Read the model definition and answer for the solid it produces. Units are mm, in the model's axes. Coordinates: 2 decimals unless noted, no trailing zeros. Loops run counter-clockwise (first coordinate to the right, second up) from the corner with the lowest first, then second, coordinate; pieces in that order, holes last. Notation, with made-up numbers: (59.5, 14.5) -> (67.5, 14.5) arc R31 ccw to (67.5, 38.5) -> close; hole circle Ø10 at (-5.5, 67.5). An arc over 180 degrees is marked (long way). Answer as CSV lines item,"result".
```python
from build123d import *

# Parameters (mm, degrees)
EXTRUDE_1_DEPTH     = 4
SKETCH_3_R          = 15
SKETCH_3_R_2        = 2.1
CUT_EXTRUDE_1_DEPTH = 4
SKETCH_4_R          = 2.15
CUT_EXTRUDE_2_DEPTH = 4
SKETCH_5_R          = 1.6
CUT_EXTRUDE_3_DEPTH = 4
EXTRUDE_2_DEPTH     = 4


with BuildPart() as part:
    # 草图2 → 凸台-拉伸1 (new body)
    with BuildSketch(Plane.XY):
        Polygon((131.137809217, 89.374251193), (132.400858097, 9.374251193), (72.408334633, 8.427082574), (71.145285753, 88.427082574), align=None)
    extrude(amount=EXTRUDE_1_DEPTH)

    # 草图3 → 切除-拉伸1 (cut)
    with BuildSketch(Plane.XY.offset(4)):
        with Locations((100.473333038, 48.885132061)):
            Circle(SKETCH_3_R)
        with Locations((119.759256959, 54.181653421)):
            Circle(SKETCH_3_R_2)
        with Locations((95.417293127, 29.53477133)):
            Circle(SKETCH_3_R_2)
        with Locations((86.243449028, 62.938971432)):
            Circle(SKETCH_3_R_2)
    extrude(amount=-CUT_EXTRUDE_1_DEPTH, mode=Mode.SUBTRACT)

    # 草图4 → 切除-拉伸2 (cut)
    with BuildSketch(Plane.XY.offset(4)):
        with Locations((77.239254962, 82.522547089)):
            Circle(SKETCH_4_R)
        with Locations((78.31271273, 14.531020496)):
            Circle(SKETCH_4_R)
    extrude(amount=-CUT_EXTRUDE_2_DEPTH, mode=Mode.SUBTRACT)

    # 草图5 → 切除-拉伸3 (cut)
    with BuildSketch(Plane.XY.offset(4)):
        with Locations((120.233896778, 83.201351266)):
            Circle(SKETCH_5_R)
        with Locations((120.423330501, 71.202846573)):
            Circle(SKETCH_5_R)
        with Locations((121.117920822, 27.208329366)):
            Circle(SKETCH_5_R)
        with Locations((121.307354546, 15.209824673)):
            Circle(SKETCH_5_R)
    extrude(amount=-CUT_EXTRUDE_3_DEPTH, mode=Mode.SUBTRACT)

    # 草图6 → 凸台-拉伸2 (add)
    with BuildSketch(Plane.XY.offset(4)):
        Polygon((132.156015483, 24.882288469), (131.934981929, 38.882288469), (135.934483494, 38.945433043), (136.155517047, 24.945433043), align=None)
        Polygon((131.603500455, 59.877927156), (131.382494444, 73.876182631), (135.381996008, 73.939327206), (135.60300202, 59.941071731), align=None)
    extrude(amount=-EXTRUDE_2_DEPTH)


solid = part.part
```
Q1. Given pin 1 Ø2.5 at (x, y) = (77.24, 82.52) entering from -Z; pin 2 Ø1 at (y, z) = (39.5, 1) entering from -X, each flat-ended and moving along its own axis, determine where each tip first touches the part or whether it passes through.
Results:
pin 1,"passes through"
pin 2,"stops at x = 71.91"
Q2. For a pull along X with two mould halves and no side action, classify faces 1 (the face through (119, 49, 0)), 2 (the face through (119.52, 27.28, 2.03)) as pulls with the +X half, pulls with the -X half, needs draft (parallel to the pull), parting line crosses it, or undercut.
Results:
face 1,"needs draft"
face 2,"undercut"
Q3. Find the intervals of material crossed by probe 1 along X at (y, z) = (53, 1.3); probe 2 along Y at (x, z) = (96.5, 3.2); probe 3 along Y at (x, z) = (95.5, 2.5), in increasing order. Write a range as [from, to].
Results:
probe 1,"x = [71.7, 86.05], [114.9, 118.02], [121.5, 131.71]"
probe 2,"y = [8.81, 27.74], [31.33, 34.42], [63.35, 88.83]"
probe 3,"y = [8.79, 27.44], [31.63, 34.73], [63.04, 88.81]"
Q4. A cutting plane is placed at A-A, the plane x = 107. Write down the section's boundary in (y, z).
Results:
outline,"(8.97, 0) -> (35.38, 0) -> (35.38, 4) -> (8.97, 4) -> close; (62.39, 0) -> (88.99, 0) -> (88.99, 4) -> (62.39, 4) -> close"
Q5. A cutting plane is placed at C-C, the plane z = 1.9. Give the number of separate pieces and of enclosed holes in the cut face, and give its area (3 significant figures).
Results:
separate pieces,"1"
enclosed holes,"10"
area,"4,100 mm²"
Q6. A cutting plane is placed at B-B, the plane y = 43. Write down the section's boundary in (x, z).
Results:
outline,"(71.86, 0) -> (86.68, 0) -> (86.68, 4) -> (71.86, 4) -> close; (114.27, 0) -> (131.87, 0) -> (131.87, 4) -> (114.27, 4) -> close"
